Autodesk Inventor part; units mm, degrees
ref_plane "YZ Plane" through (0, 0, 0) normal (1, 0, 0) x (0, 1, 0)
ref_plane "XZ Plane" through (0, 0, 0) normal (0, 1, 0) x (-1, 0, 0)
ref_plane "XY Plane" through (0, 0, 0) normal (0, 0, 1) x (1, 0, 0)
sketch "Sketch1" plane through (0, 0, 0) normal (1, 0, 0) x (0, 1, 0)
  line L0 (0, 0) -> (0, -6.5)
  line L1 (0, -6.5) -> (2, -6.5)
  line L2 (2, -6.5) -> (4.16, -17.286)
  line L3 (0, 0) -> (2, 0)
  line L4 (2, 0) -> (5.4115, -17.0354)
  line L5 (5.4115, -17.0354) -> (4.16, -17.286)
  dimension "d0" = 6.5
  dimension "d1" = 2
  dimension "d2" = 10.786
  dimension "d3" = 2.16
extrude "Extrusion1" add sketch "Sketch1" along normal blind 50
sketch "Sketch2" plane through (50, 0, 0) normal (1, 0, 0) x (0, 0, -1)
  line L0 (0, 0) -> (6.5, 0)
  line L1 (6.5, 0) -> (6.5, 2)
  line L2 (6.5, 2) -> (17.286, 4.16)
  line L3 (17.286, 4.16) -> (17.0354, 5.4115)
  line L4 (17.0354, 5.4115) -> (0, 2)
  line L5 (0, 2) -> (0, 0)
  line L6 (8.7683, 2.4543) -> (8.5177, 3.7057)
extrude "Extrusion2" add sketch "Sketch2" along normal blind 50 contours L4 L3 L2 L6
sketch "Sketch3" plane through (100, 0, 0) normal (1, 0, 0) x (0, 0, -1)
  line L0 (8.7683, 2.4543) -> (8.5177, 3.7057)
  line L1 (8.5177, 3.7057) -> (0, 2)
  line L2 (0, 2) -> (0, 0)
  line L3 (0, 0) -> (6.5, 0)
  line L4 (6.5, 0) -> (6.5, 2)
  line L5 (6.5, 2) -> (8.7683, 2.4543)
  line L6 (17.0354, 5.4115) -> (8.5177, 3.7057)
  line L7 (8.5177, 3.7057) -> (8.7683, 2.4543)
  line L8 (8.7683, 2.4543) -> (17.286, 4.16)
  line L9 (17.286, 4.16) -> (17.0354, 5.4115)
extrude "Extrusion3" add sketch "Sketch3" along normal blind 50
sketch "Sketch4" plane through (100, 0, -6.5) normal (0, -1, 0) x (1, 0, 0)
  circle A0 centre (-85, 3.25) radius 1.55
  circle A1 centre (-62.5, 3.25) radius 1.55
  line L0 (-100, 6.5) -> (-100, 0)
  line L1 (-100, 6.5) -> (-50, 6.5)
  circle A2 centre (35, 3.25) radius 1.55
  circle A3 centre (12.5, 3.25) radius 1.55
  line L2 (0, 6.5) -> (50, 6.5)
  line L3 (50, 6.5) -> (50, 0)
  point P0 (-100, 3.25)
  dimension "d10" = 37.5
  dimension "d11" = 15
  dimension "d12" = 3.25
  dimension "d13" = 3.1
  dimension "d14" = 3.25
  dimension "d15" = 3.1
  dimension "d16" = 3.1
  dimension "d17" = 3.1
  dimension "d18" = 3.25
  dimension "d19" = 3.25
  dimension "d20" = 15
  dimension "d21" = 37.5
extrude "Extrusion4" cut sketch "Sketch4" against normal blind 3
sketch "Sketch5" plane through (150, 0, 0) normal (1, 0, 0) x (0, 0, -1)
  line L0 (0, 0) -> (13.9221, 9.3906)
  line L1 (0, 0) -> (16.7931, 0) construction
  line L2 (0, 0) -> (4.2172, 2.8445)
  line L3 (1.7, 2.3404) -> (4.8, 2.9612)
  line L4 (17.0354, 5.4115) -> (0, 2)
  line L5 (0, 2) -> (4.2172, 2.8445)
  line L6 (0, 2) -> (0, 0)
  dimension "d24" = 34
extrude "Extrusion5" cut sketch "Sketch5" against normal blind 150
sketch "Sketch6" plane through (150, 0, 0) normal (1, 0, 0) x (0, 0, -1)
  line L0 (0, 0) -> (6.5, 0)
  line L1 (6.5, 0) -> (10.7172, 2.8445)
  line L2 (6.5, 2) -> (8.7683, 2.4543)
  line L3 (4.2172, 2.8445) -> (0, 0)
  line L4 (6.5, 0) -> (6.5, 2)
  line L5 (10.7172, 2.8445) -> (6.5, 2)
extrude "Extrusion6" add sketch "Sketch6" against normal blind 50
sketch "Sketch7" plane through (0, 0, 0) normal (-1, 0, 0) x (0, 0, 1)
  line L0 (0, 0) -> (-4.2172, 2.8445)
  line L1 (-8.5177, 3.7057) -> (-4.2172, 2.8445)
  line L2 (-8.5177, 3.7057) -> (-8.7683, 2.4543)
  line L3 (-10.7172, 2.8445) -> (-8.7683, 2.4543)
  line L4 (-10.7172, 2.8445) -> (-6.5, 0)
  line L5 (0, 0) -> (-6.5, 0)
  line L6 (-6.5, 2) -> (-17.286, 4.16)
  line L7 (-6.5, 0) -> (-6.5, 2)
  line L8 (-10.7172, 2.8445) -> (-6.5, 0)
extrude "Extrusion7" add sketch "Sketch7" against normal blind 50 contours L4 L3 L6 L7
properties part number "przod"
Can you work these out from the model? Positions are in its coordinate system, mm. Coordinates: 2 decimals unless noted, no trailing zeros. Loops run counter-clockwise (first coordinate to the right, second up) from the corner with the lowest first, then second, coordinate; pieces in that order, holes last.
1) Imagine slicing it at D-D on x = 135. List the corners of the cut face in (y, z) for me.
2) Imagine slicing it at A-A on x = 37.5. List the corners of the cut face in (y, z) for me.
3) Imagine slicing it at C-C on x = 107.5. List the corners of the cut face in (y, z) for me.
4) For pin 1 (1.5 mm diameter, centred on x = 62.5, z = -11, fed in from +Y); pin 2 (3 mm diameter, centred on x = 77.5, z = -11.5, fed in from +Y); pin 3 (5 mm diameter, centred on x = 80, z = -12.5, fed in from +Y), each with a flat end and sliding along its axis, tell me the tip position at first contact or that it passes through.
5) Imagine slicing it at B-B on z = -15.75. List the corners of the cut face in (x, y) for me.
6) Thinking about a two-plate mould opening in Z: for faces 1 (the flat face through (24.65, 1.442, -8.638)), 2 (the flat face through (0, 3, -8)), 3 (the cylindrical face through (112.164, 1.131, -4.763)), 4 (the flat face through (25.35, 1.402, -2.079)), which applies, pulls with the +Z half, pulls with the -Z half, needs draft (parallel to the pull), parting line crosses it, or undercut?
7) I need wall thicknesses on probe 1 along X at (y, z) = (2.15, -3.25); probe 2 along Z at (x, y) = (116, 1.15); probe 3 along Y at (x, z) = (15, -13). Which ranges of each line are inside material? Lowest first, please.
Completed:
1. outline: (0, -6.5) - (2.84, -10.72) - (4.16, -17.29) - (5.41, -17.04) - (3.71, -8.52) - (2.96, -4.8) - (0, -4.8) - close; (0, -1.7) - (1.15, -1.7) - (0, 0) - close
2. outline: (0, -6.5) - (2.84, -10.72) - (4.16, -17.29) - (5.41, -17.04) - (2.96, -4.8) - (0, -4.8) - close; (0, -1.7) - (1.15, -1.7) - (0, 0) - close
3. outline: (0, -6.5) - (2.84, -10.72) - (4.16, -17.29) - (5.41, -17.04) - (3.71, -8.52) - (2.84, -4.22) - (0, 0) - close
4. pin 1: stops at y = 4.35
4. pin 2: stops at y = 4.6
4. pin 3: stops at y = 5
5. outline: (0, 3.85) - (150, 3.85) - (150, 5.15) - (0, 5.15) - close
6. face 1: pulls with the -Z half
6. face 2: needs draft
6. face 3: undercut
6. face 4: pulls with the +Z half
7. probe 1: x = 0 to 13.45, 16.55 to 35.95, 39.05 to 50, 100 to 110.95, 114.05 to 133.45, 136.55 to 150
7. probe 2: z = -8.2 to -1.7
7. probe 3: y = 3.3 to 4.6
